from build123d import *

# Parameters (mm, degrees)
F1_DEPTH = 6.35
F3_DEPTH = 25.4
F5_DEPTH = 25.4


with BuildPart() as f1:
    # F0 (on Top) → F1 (new body)
    with BuildSketch(Plane.XY):
        with BuildLine():
            Line((113.9825, 84.1375), (-113.9825, 84.1375))
            ThreePointArc((-113.9825, 84.1375), (-117.574602, 82.649602), (-119.0625, 79.0575))
            Line((-119.0625, 79.0575), (-119.0625, -79.0575))
            ThreePointArc((-119.0625, -79.0575), (-117.574602, -82.649602), (-113.9825, -84.1375))
            Line((-113.9825, -84.1375), (113.9825, -84.1375))
            ThreePointArc((113.9825, -84.1375), (117.574602, -82.649602), (119.0625, -79.0575))
            Line((119.0625, -79.0575), (119.0625, 79.0575))
            ThreePointArc((119.0625, 79.0575), (117.574602, 82.649602), (113.9825, 84.1375))
        make_face()
    extrude(amount=F1_DEPTH)

    # F2 (on face) → F3 (cut)
    with BuildSketch(Plane.XY.offset(6.35)):
        Polygon((22.479, 70.448201), (0, 70.448201), (-22.479, 70.448201), (-22.479, -19.467799), (-68.098701, -65.0875), (0, -65.0875), (68.098701, -65.0875), (22.479, -19.467799), align=None)
    extrude(amount=-F3_DEPTH, mode=Mode.SUBTRACT)

    # F4 (on face) → F5 (cut)
    with BuildSketch(Plane.XY.offset(6.35)):
        with BuildLine():
            ThreePointArc((-22.9616, 71.718201), (-23.518376, 71.487577), (-23.749, 70.930801))
            Line((-23.749, 70.930801), (-23.749, -18.615596))
            ThreePointArc((-23.749, -18.615596), (-23.808937, -18.916921), (-23.979624, -19.172372))
            Line((-23.979624, -19.172372), (-69.820576, -65.013324))
            ThreePointArc((-69.820576, -65.013324), (-69.991263, -65.871425), (-69.263801, -66.3575))
            Line((-69.263801, -66.3575), (69.263801, -66.3575))
            ThreePointArc((69.263801, -66.3575), (69.991263, -65.871425), (69.820576, -65.013324))
            Line((69.820576, -65.013324), (23.979624, -19.172372))
            ThreePointArc((23.979624, -19.172372), (23.808937, -18.916921), (23.749, -18.615596))
            Line((23.749, -18.615596), (23.749, 70.930801))
            ThreePointArc((23.749, 70.930801), (23.518376, 71.487577), (22.9616, 71.718201))
            Line((22.9616, 71.718201), (-22.9616, 71.718201))
        make_face()
    extrude(amount=-F5_DEPTH, mode=Mode.SUBTRACT)


solid = f1.part
Geometry check sheet. Reference: the model listing, model coordinates, mm. A direction names the side the tool comes from. Give positions to 0.01 mm unless a question says otherwise; leave off trailing zeros. Loops run counter-clockwise (first coordinate to the right, second up) from the corner with the lowest first, then second, coordinate; pieces in that order, holes last. Notation, with made-up numbers: M 46,47 L 82,47 A32 cw 82,84 Z; hole C 79.25,-6 d10. An arc over 180 degrees is marked long. Answer as a JSON object with one key per item and string values. Group by question number.
Item 1: Access from +Z, -Z, +X, -X, +Y, -Y to the whole of each face (thin tool, end or side, straight path). Record for faces 4 (the flat face through (23.749, 26, 3)), 5 (the flat face through (25, 1, 6.35)).
Item 2: Mould release check, pull along X, two halves, no side actions. Record for faces 1 (the flat face through (25, 1, 0)), 2 (the cylindrical face through (117.535, -82.689, 3.131)), 3 (the flat face through (-23.749, 27, 3)): pulls with the +X half, pulls with the -X half, needs draft (parallel to the pull), parting line crosses it, or undercut.
Item 3: Sectioned sample at A-A on x = 12.5. Record the boundary of the cut face in (y, z).
Item 4: Sectioned sample at C-C on z = 4.25. Record the boundary of the cut face in (x, y).
Item 5: Material ranges on L1, parallel to Y at x = -21.5, z = 1.5; L2, parallel to X at y = -9.5, z = 1.25; L3, parallel to Y at x = -29, z = 1.5, recorded low to high.
Item 6: Gauge pin test, flat end, axial feed: pin 1 (4 mm diameter, centred on x = 28, y = -19, fed in from -Z). Record the tip position at first contact, or that the pin passes through.
Item 7: Sectioned sample at B-B on y = -10. Record the boundary of the cut face in (x, z), plus the area to 3 significant figures.
Findings below:
{
 "1": {"face 4": "+Z, -Z", "face 5": "+Z, +X, -X, +Y, -Y"},
 "2": {"face 1": "needs draft", "face 2": "pulls with the +X half", "face 3": "undercut"},
 "3": {"outline": "M -84.14,0 L -66.36,0 L -66.36,6.35 L -84.14,6.35 Z; M 71.72,0 L 84.14,0 L 84.14,6.35 L 71.72,6.35 Z"},
 "4": {"outline": "M -119.06,-79.06 A5.08 ccw -113.98,-84.14 L 113.98,-84.14 A5.08 ccw 119.06,-79.06 L 119.06,79.06 A5.08 ccw 113.98,84.14 L -113.98,84.14 A5.08 ccw -119.06,79.06 Z; hole M -69.82,-65.01 A0.79 ccw -69.26,-66.36 L 69.26,-66.36 A0.79 ccw 69.82,-65.01 L 23.98,-19.17 A0.79 cw 23.75,-18.62 L 23.75,70.93 A0.79 ccw 22.96,71.72 L -22.96,71.72 A0.79 ccw -23.75,70.93 L -23.75,-18.62 A0.79 cw -23.98,-19.17 Z"},
 "5": {"L1": "-84.14 to -66.36, 71.72 to 84.14", "L2": "-119.06 to -23.75, 23.75 to 119.06", "L3": "-84.14 to -66.36, -24.19 to 84.14"},
 "6": {"pin 1": "z = 0"},
 "7": {"outline": "M -119.06,0 L -23.75,0 L -23.75,6.35 L -119.06,6.35 Z; M 23.75,0 L 119.06,0 L 119.06,6.35 L 23.75,6.35 Z", "area": "1,210 mm2"}
}
